from build123d import *

# Parameters (mm, degrees)
SKETCH1_W           = 3
SKETCH1_H           = 2.91365756
BOSS_EXTRUDE1_DEPTH = 3


with BuildPart() as part:
    # Sketch1 → Boss-Extrude1 (new body)
    with BuildSketch(Plane(origin=(0, 0, 0), x_dir=(1, 0, 0), z_dir=(0, 1, 0))):
        with BuildLine():
            Line((-8, -45.8), (-11.857864376, -45.8))
            ThreePointArc((-11.857864376, -45.8), (-15.6846987, -45.038795325), (-18.928932188, -42.871067812))
            Line((-18.928932188, -42.871067812), (-20.571067812, -41.228932188))
            ThreePointArc((-20.571067812, -41.228932188), (-23.8153013, -39.061204675), (-27.642135624, -38.3))
            Line((-27.642135624, -38.3), (-35.353653112, -38.3))
            ThreePointArc((-35.353653112, -38.3), (-37.452206123, -38.077324545), (-39.457299885, -37.419215052))
            Line((-39.457299885, -37.419215052), (-42.320729355, -36.13067179))
            ThreePointArc((-42.320729355, -36.13067179), (-43.179502711, -35.392771065), (-43.5, -34.30682878))
            Line((-43.5, -34.30682878), (-43.5, -31.39317122))
            ThreePointArc((-43.5, -31.39317122), (-43.179502711, -30.307228935), (-42.320729355, -29.56932821))
            Line((-42.320729355, -29.56932821), (-39.457299885, -28.280784948))
            ThreePointArc((-39.457299885, -28.280784948), (-37.452206123, -27.622675455), (-35.353653112, -27.4))
            Line((-35.353653112, -27.4), (-27.642135624, -27.4))
            ThreePointArc((-27.642135624, -27.4), (-23.8153013, -26.638795325), (-20.571067812, -24.471067812))
            Line((-20.571067812, -24.471067812), (-18.928932188, -22.828932188))
            ThreePointArc((-18.928932188, -22.828932188), (-15.6846987, -20.661204675), (-11.857864376, -19.9))
            Line((-11.857864376, -19.9), (-8, -19.9))
            Line((-8, -19.9), (-8, -3))
            Line((-8, -3), (-3, -3))
            Line((-3, -3), (-3, 0))
            Line((-3, 0), (0, 0))
            Line((0, 0), (0, -65.7))
            Line((0, -65.7), (-3, -65.7))
            Line((-3, -65.7), (-3, -62.7))
            Line((-3, -62.7), (-8, -62.7))
            Line((-8, -62.7), (-8, -45.8))
        make_face()
        with Locations((-40, -32.85)):
            Rectangle(SKETCH1_W, SKETCH1_H, mode=Mode.SUBTRACT)
    extrude(amount=BOSS_EXTRUDE1_DEPTH)


solid = part.part
Verification items for the finished model (mm, model axes). A direction names the side the tool comes from. Give positions to 0.01 mm unless a question says otherwise; leave off trailing zeros. Write each loop counter-clockwise with the first axis right and the second up, starting at its lowest first coordinate (ties: lowest second). Pieces come first, ordered by that corner, then holes. Notation, with made-up numbers: (89, 65) -> (125, 65) arc R19 ccw to (125, 101) -> close; hole circle Ø9 at (-1, -4). An arc over 180 degrees is marked (long way). Use CSV: the item, a comma, the result in double quotes.
(1) Sectioned sample at D-D (z = 6). Record the cut outline in (x, y).
Derived:
outline,"(-8, 0) -> (0, 0) -> (0, 3) -> (-8, 3) -> close"
(2) Set-up check for faces 1 (the flat face through (-6, 1, 3)), 2 (the flat face through (-3, 1, 64)), 3 (the flat face through (-2, 1, 0)): record each of +Z, -Z, +X, -X, +Y, -Y from which the full face is reachable in a straight line by a thin tool's end or side.
Derived:
face 1,"-Z, -X, +Y, -Y"
face 2,"+Z, -X, +Y, -Y"
face 3,"-Z, +X, -X, +Y, -Y"
(3) Sectioned sample at C-C (x = -4). Record the cut outline in (y, z), plus the area to 3 significant figures.
Derived:
outline,"(0, 3) -> (3, 3) -> (3, 62.7) -> (0, 62.7) -> close"
area,"179 mm^2"
(4) Sectioned sample at A-A (z = 33). Record the cut outline in (x, y).
Derived:
outline,"(-43.5, 0) -> (-41.5, 0) -> (-41.5, 3) -> (-43.5, 3) -> close; (-38.5, 0) -> (0, 0) -> (0, 3) -> (-38.5, 3) -> close"
(5) Release check for a two-part mould opening along Z. For faces 4 (the flat face through (-40, 1, 31.393)), 5 (the flat face through (-8, 1, 12)), 6 (the flat face through (-40.869, 1.479, 36.784)), 7 (the flat face through (-40, 1, 34.307)) record: +Z half, -Z half, draft (parallel to the pull), parting line (faces both ways), or undercut.
Derived:
face 4,"undercut"
face 5,"draft"
face 6,"+Z half"
face 7,"undercut"
(6) Go/stop test with flat-tipped pins: pin 1 (1 mm diameter, centred on y = 0.5, z = 36, fed in from +X); pin 2 (0.9 mm diameter, centred on x = -6.5, y = 2, fed in from +Z); pin 3 (1.5 mm diameter, centred on y = 2, z = 52.5, fed in from -X); pin 4 (1.5 mm diameter, centred on y = 1, z = 1, fed in from -X). Record where each tip stops, or that it passes through.
Derived:
pin 1,"stops at x = 0"
pin 2,"stops at z = 62.7"
pin 3,"stops at x = -8"
pin 4,"stops at x = -3"
(7) Material ranges on L1, parallel to X at y = 2.5, z = 17.5; L2, parallel to Z at x = -11, y = 0.65; L3, parallel to Z at x = -6, y = 1.35, recorded low to high.
Derived:
L1,"x = -8 to 0"
L2,"z = 19.9 to 45.8"
L3,"z = 3 to 62.7"
